Check sheet for the modelled part. Datum: model origin and axes. Units: mm. A direction names the side the tool comes from. Round coordinates to 2 decimals unless told otherwise and drop trailing zeros. Loops run counter-clockwise (first coordinate to the right, second up) from the corner with the lowest first, then second, coordinate; pieces in that order, holes last. Notation, with made-up numbers: M 22.5,60.25 L 44.5,60.25 A18 cw 44.5,69.25 Z; hole C 39.25,46 d11. An arc over 180 degrees is marked long. Write item = value, one per line. Start each with the question number.
(1) Cross-section at D-D on z = 18.25. Record the boundary of the cut face in (x, y).
(2) Go/stop test with flat-tipped pins: P1, Ø12, axis at x = 6.5, y = -5, coming from the +Z side; P2, Ø7, axis at x = -10.83, y = 6.25, coming from the +Z side; P3, Ø10, axis at y = -6, z = 4.5, coming from the -X side; P4, Ø3, axis at x = -10, y = -7, coming from the -Z side. Record where each tip stops, or that it passes through.
(3) Cross-section at B-B on y = 0. Record the boundary of the cut face in (x, z).
(4) Mould release check, pull along Z, two halves, no side actions. Record for faces 1 (the face through (-11, 6, 8)), 2 (the face through (-0.1, -19.2, 26)), 3 (the face through (-15.99, 14.67, 26.99)): pulls with the +Z half, pulls with the -Z half, needs draft (parallel to the pull), parting line crosses it, or undercut.
(5) Set-up check for faces 4 (the face through (11, -6, 8)), 5 (the face through (-0.1, 19.2, 0)), 6 (the face through (0, 4, 13)), 7 (the face through (5, 15, 28)), 8 (the face through (-3, 0, 6)): record each of +Z, -Z, +X, -X, +Y, -Y from which the full face is reachable in a straight line by a thin tool's end or side.
(6) Scan lines: L1, parallel to Y at x = 0, z = 7.25; L2, parallel to Y at x = -11, z = 2; L3, parallel to X at y = 0.5, z = 25.5. Record each from-to range of solid material in increasing order. Write a range as from..to.
(7) Cross-section at C-C on z = 0.75. Record the boundary of the cut face in (x, y), plus the area to 3 significant figures.
(8) Cross-section at A-A on x = 0. Record the boundary of the cut face in (y, z), plus the area to 3 significant figures.
from build123d import *

# Parameters (mm, degrees)
CROQUIS2_R              = 19
SALIENTE_EXTRUIR1_DEPTH = 26
CROQUIS3_R              = 21.7
SALIENTE_EXTRUIR2_DEPTH = 2
SALIENTE_EXTRUIR3_START = 2
CROQUIS4_R              = 21.7
SALIENTE_EXTRUIR3_DEPTH = 2
CROQUIS5_R              = 15
CORTAR_EXTRUIR1_DEPTH   = 15
CROQUIS6_R              = 3
CORTAR_EXTRUIR2_DEPTH   = 35.158161543
CROQUIS7_R              = 3
CORTAR_EXTRUIR3_DEPTH   = 10


with BuildPart() as part:
    # Croquis2 → Saliente-Extruir1 (new body)
    with BuildSketch(Plane.XY):
        with Locations(Location((0, 0, 0), (0, 0, 180))):
            Circle(CROQUIS2_R)
    extrude(amount=SALIENTE_EXTRUIR1_DEPTH)

    # Croquis3 → Saliente-Extruir2 (add)
    with BuildSketch(Plane.XY.offset(26)):
        Circle(CROQUIS3_R)
    extrude(amount=SALIENTE_EXTRUIR2_DEPTH)

    # Croquis4 → Saliente-Extruir3 (add)
    with BuildSketch(Plane(origin=(0, 0, 0), x_dir=(-1, 0, 0), z_dir=(0, 0, -1)).offset(SALIENTE_EXTRUIR3_START)):
        with Locations(Location((0, 0, 0), (0, 0, 180))):
            Circle(CROQUIS4_R)
    extrude(amount=-SALIENTE_EXTRUIR3_DEPTH)

    # Croquis5 → Cortar-Extruir1 (cut)
    with BuildSketch(Plane.XY.offset(28)):
        Circle(CROQUIS5_R)
    extrude(amount=-CORTAR_EXTRUIR1_DEPTH, mode=Mode.SUBTRACT)

    # Croquis6 → Cortar-Extruir2 (cut, through all)
    with BuildSketch(Plane.XY.offset(13)):
        Circle(CROQUIS6_R)
    extrude(amount=-CORTAR_EXTRUIR2_DEPTH, mode=Mode.SUBTRACT)

    # Croquis7 → Cortar-Extruir3 (cut)
    with BuildSketch(Plane(origin=(0, 0, -2), x_dir=(-1, 0, 0), z_dir=(0, 0, -1))):
        with Locations((0, 12.5)):
            Circle(CROQUIS7_R)
        with Locations((10.825317547, 6.25)):
            Circle(CROQUIS7_R)
        with Locations((10.825317547, -6.25)):
            Circle(CROQUIS7_R)
        with Locations((0, -12.5)):
            Circle(CROQUIS7_R)
        with Locations((-10.825317547, -6.25)):
            Circle(CROQUIS7_R)
        with Locations((-10.825317547, 6.25)):
            Circle(CROQUIS7_R)
    extrude(amount=-CORTAR_EXTRUIR3_DEPTH, mode=Mode.SUBTRACT)


solid = part.part
Result:
q1.outline = C 0,0 d38; hole C 0,0 d30
q2.P1 = 13
q2.P2 = 28
q2.P3 = -21.36
q2.P4 = 8
q3.outline = M -21.7,-2 L -3,-2 L -3,13 L -15,13 L -15,28 L -21.7,28 L -21.7,26 L -19,26 L -19,0 L -21.7,0 Z; M 3,-2 L 21.7,-2 L 21.7,0 L 19,0 L 19,26 L 21.7,26 L 21.7,28 L 15,28 L 15,13 L 3,13 Z
q4.face_1 = pulls with the -Z half
q4.face_2 = undercut
q4.face_3 = needs draft
q5.face_4 = -Z
q5.face_5 = none
q5.face_6 = +Z
q5.face_7 = +Z, +X, -X, +Y, -Y
q5.face_8 = +Z, -Z
q6.L1 = -19..-15.5, -9.5..-3, 3..9.5, 15.5..19
q6.L2 = -15.49..-9.24, -3.26..3.26, 9.24..15.49
q6.L3 = -18.99..-14.99, 14.99..18.99
q7.outline = C 0,0 d38; hole C -10.83,-6.25 d6; hole C -10.83,6.25 d6; hole C 0,-12.5 d6; hole C 0,0 d6; hole C 0,12.5 d6; hole C 10.83,-6.25 d6; hole C 10.83,6.25 d6
q7.area = 936 mm^2
q8.outline = M -21.7,-2 L -15.5,-2 L -15.5,8 L -9.5,8 L -9.5,-2 L -3,-2 L -3,13 L -15,13 L -15,28 L -21.7,28 L -21.7,26 L -19,26 L -19,0 L -21.7,0 Z; M 3,-2 L 9.5,-2 L 9.5,8 L 15.5,8 L 15.5,-2 L 21.7,-2 L 21.7,0 L 19,0 L 19,26 L 21.7,26 L 21.7,28 L 15,28 L 15,13 L 3,13 Z
q8.area = 502 mm^2
